Print and shaded views of the part. All mm, measured from the part's lowest x, y and z. A direction names the side the tool comes from. Round coordinates to 2 decimals unless told otherwise and drop trailing zeros. Loops run counter-clockwise (first coordinate to the right, second up) from the corner with the lowest first, then second, coordinate; pieces in that order, holes last. Notation, with made-up numbers: (-5, 82) -> (20, 82) arc R27 cw to (20, 102) -> close; hole circle Ø8 at (-28, 61.5). An arc over 180 degrees is marked (long way). Use a Markdown table: item, result.
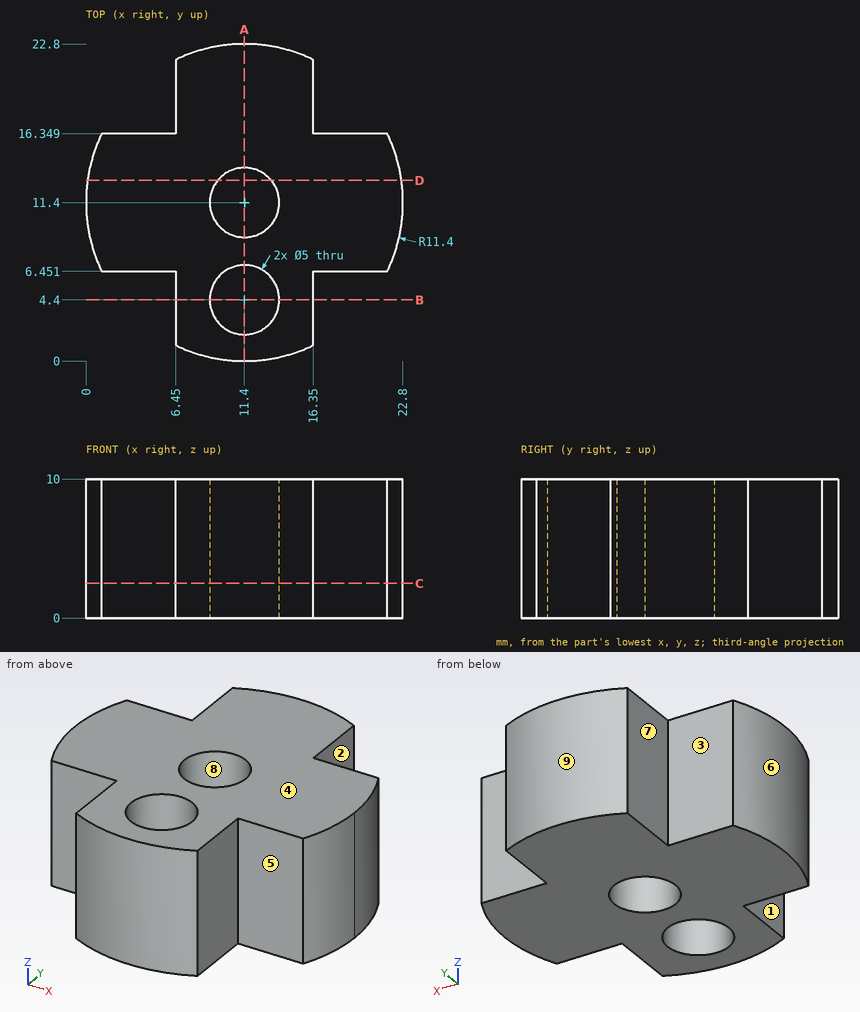
Q1. Tool access for the marked faces 1, 2, 3, 4 and 5: list every direction of +Z, -Z, +X, -X, +Y, -Y with a clear straight run to the whole face (end or side of a thin tool).
Results list:
| item | result |
|---|---|
| face 1 | +Z, -Z, -X, -Y |
| face 2 | +Z, -Z, +X, +Y |
| face 3 | +Z, -Z, -X, +Y |
| face 4 | +Z, +X, -X, +Y, -Y |
| face 5 | +Z, -Z, +X, -Y |
Q2. Band-saw the part on D-D, the plane y = 13. Give the cut face in (x, z), plus the area to 3 significant figures.
Results list:
| item | result |
|---|---|
| outline | (0.11, 0) -> (9.48, 0) -> (9.48, 10) -> (0.11, 10) -> close; (13.32, 0) -> (22.69, 0) -> (22.69, 10) -> (13.32, 10) -> close |
| area | 187 mm² |
Q3. Drill centre lines: L1, parallel to Y at x = 11.4, z = 3; L2, parallel to Y at x = 12.25, z = 5.25; L3, parallel to X at y = 16.5, z = 9.25. Where is each one in solid material? Low to high. Write a range as from..to.
Results list:
| item | result |
|---|---|
| L1 | y = 0..1.9, 6.9..8.9, 13.9..22.8 |
| L2 | y = 0.03..2.05, 6.75..9.05, 13.75..22.77 |
| L3 | x = 6.45..16.35 |
Q4. Band-saw the part on A-A, the plane x = 11.4. Give the cut face in (y, z), plus the area to 3 significant figures.
Results list:
| item | result |
|---|---|
| outline | (0, 0) -> (1.9, 0) -> (1.9, 10) -> (0, 10) -> close; (6.9, 0) -> (8.9, 0) -> (8.9, 10) -> (6.9, 10) -> close; (13.9, 0) -> (22.8, 0) -> (22.8, 10) -> (13.9, 10) -> close |
| area | 128 mm² |
Q5. Flat gauge pins, fed straight in: pin 1 (2.5 mm diameter, centred on x = 3.5, z = 7, fed in from +Y); pin 2 (6 mm diameter, centred on y = 4.5, z = 5, fed in from +X); pin 3 (6 mm diameter, centred on y = 12.5, z = 3.5, fed in from -X); pin 4 (1.6 mm diameter, centred on y = 4, z = 6.5, fed in from -X). Where does each tip first touch, or does it go through?
Results list:
| item | result |
|---|---|
| pin 1 | stops at y = 16.35 |
| pin 2 | stops at x = 22.11 |
| pin 3 | stops at x = 0 |
| pin 4 | stops at x = 6.45 |
Q6. Pull direction Y, two halves, no side cores. Call the marked faces 6, 7, 8 and 9: released by +Y, released by -Y, zero draft, split by the parting line, or undercut.
Results list:
| item | result |
|---|---|
| face 6 | split by the parting line |
| face 7 | zero draft |
| face 8 | undercut |
| face 9 | released by +Y |
Q7. Band-saw the part on C-C, the plane z = 2.5. Give the cut face in (x, y).
Results list:
| item | result |
|---|---|
| outline | (1.13, 6.45) -> (6.45, 6.45) -> (6.45, 1.13) arc R11.4 ccw to (16.35, 1.13) -> (16.35, 6.45) -> (21.67, 6.45) arc R11.4 ccw to (22.8, 11.4) arc R11.4 ccw to (21.67, 16.35) -> (16.35, 16.35) -> (16.35, 21.67) arc R11.4 ccw to (6.45, 21.67) -> (6.45, 16.35) -> (1.13, 16.35) arc R11.4 ccw to start; hole circle Ø5 at (11.4, 4.4); hole circle Ø5 at (11.4, 11.4) |
Q8. Band-saw the part on B-B, the plane y = 4.4. Give the cut face in (x, z), plus the area to 3 significant figures.
Results list:
| item | result |
|---|---|
| outline | (6.45, 0) -> (8.9, 0) -> (8.9, 10) -> (6.45, 10) -> close; (13.9, 0) -> (16.35, 0) -> (16.35, 10) -> (13.9, 10) -> close |
| area | 49.0 mm² |
